from build123d import *


with BuildPart() as f1:
    # F0 (on Top) → F1 (revolve)
    with BuildSketch(Plane.XY):
        Polygon((74.900694, 23.233382), (45.905843, 23.233382), (45.905843, 38.353771), (15.265487, 38.353771), (15.265487, 48.903458), (0, 48.903458), (0, 38.353771), (0, 11.005023), (45.905843, 11.005023), (74.900694, 11.005023), align=None)
        Polygon((-45.905843, 11.005023), (0, 11.005023), (0, 38.353771), (0, 48.903458), (-15.265487, 48.903458), (-15.265487, 38.353771), (-45.905843, 38.353771), (-45.905843, 23.233382), (-74.900694, 23.233382), (-74.900694, 11.005023), align=None)
    revolve(axis=Axis((-0.145569, 0, 0), (1, 0, 0)))


solid = f1.part
Design review of the part built by this model. Coordinates are the model's own, in mm. A direction names the side the tool comes from. Coordinates: 2 decimals unless noted, no trailing zeros. Order: outer loops, then holes, each group sorted by start corner. A loop starts at its lowest first (then second) coordinate and runs counter-clockwise, first axis right, second up. Notation, with made-up numbers: (86, 13.5) - (109, 13.5) arc R15 cw to (109, 41.5) - close; hole circle Ø1 at (30.5, -4.5). An arc over 180 degrees is marked (long way). Put each result on its own line as item: value.
1) Insertion check: P1, Ø10, axis at x = -54, z = -28.5, coming from the +Y side; P2, Ø12, axis at x = -19, z = -33.5, coming from the +Y side; P3, Ø4, axis at y = -36.5, z = -28, coming from the +X side; P4, Ø1, axis at x = -17.5, y = -4.5, coming from the +Z side. Each pin has a flat end and moves straight along its axis. Give the tip position at first contact, or say it passes through.
Response values:
P1: passes through
P2: stops at y = 39.52
P3: stops at x = 15.27
P4: stops at z = 38.14
2) The part is to be moulded in two halves that separate along Y. For faces 1 (the face through (74.901, -5, -10)), 2 (the face through (1.049, -2.386, -10.743)), 3 (the face through (30.371, -8.314, -37.442)), say which applies: released by +Y, released by -Y, zero draft, split by the parting line, or undercut.
Response values:
face 1: zero draft
face 2: undercut
face 3: split by the parting line
3) Take a section at C-C, the plane x = -11.5. Give the boundary of the cut face in (y, z), and give its area (3 significant figures).
Response values:
outline: circle Ø97.81 at (0, 0); hole circle Ø22.01 at (0, 0)
area: 7,130 mm²
4) Tool access review of faces 4 (the face through (60.2, -3.025, 23.036)), 5 (the face through (-45.906, 17, -17)), 6 (the face through (-74.901, 5, -10)): name each direction out of +Z, -Z, +X, -X, +Y, -Y from which nothing blocks a thin tool from reaching the whole face with its end or side.
Response values:
face 4: +X
face 5: -X
face 6: +Z, -Z, -X, +Y, -Y
5) Take a section at A-A, the plane y = 0. Give the boundary of the cut face in (x, z), and give its area (3 significant figures).
Response values:
outline: (-74.9, -23.23) - (-45.91, -23.23) - (-45.91, -38.35) - (-15.27, -38.35) - (-15.27, -48.9) - (15.27, -48.9) - (15.27, -38.35) - (45.91, -38.35) - (45.91, -23.23) - (74.9, -23.23) - (74.9, -11.01) - (-74.9, -11.01) - close; (-74.9, 11.01) - (74.9, 11.01) - (74.9, 23.23) - (45.91, 23.23) - (45.91, 38.35) - (15.27, 38.35) - (15.27, 48.9) - (-15.27, 48.9) - (-15.27, 38.35) - (-45.91, 38.35) - (-45.91, 23.23) - (-74.9, 23.23) - close
area: 7,080 mm²
6) Wall thickness on L1, parallel to Z at x = 35, y = 0; L2, parallel to Z at x = -5, y = 0; L3, parallel to X at y = 20, z = 28.5: over which ranges is each line inside the solid? List them lowest first. Write a range as from..to.
Response values:
L1: z = -38.35..-11.01, 11.01..38.35
L2: z = -48.9..-11.01, 11.01..48.9
L3: x = -45.91..45.91
7) Take a section at D-D, the plane z = 29. Give the boundary of the cut face in (x, y), and give its area (3 significant figures).
Response values:
outline: (-45.91, -25.1) - (-15.27, -25.1) - (-15.27, -39.38) - (15.27, -39.38) - (15.27, -25.1) - (45.91, -25.1) - (45.91, 25.1) - (15.27, 25.1) - (15.27, 39.38) - (-15.27, 39.38) - (-15.27, 25.1) - (-45.91, 25.1) - close
area: 5,480 mm²
